Geometry check sheet. Reference: the model listing, model coordinates, mm. A direction names the side the tool comes from. Round coordinates to 2 decimals unless told otherwise and drop trailing zeros. Order: outer loops, then holes, each group sorted by start corner. A loop starts at its lowest first (then second) coordinate and runs counter-clockwise, first axis right, second up. Notation, with made-up numbers: (6, -12) - (54, -12) arc R26 ccw to (54, 19) - close; hole circle Ø1 at (28, 23). An arc over 180 degrees is marked (long way). Return JSON: item names as keys, results as strings. Group by question number.
Q1. Tool access check on faces 1 (the cylindrical face through (-36.39, -0.89, 4.93)), 2 (the cylindrical face through (24.245, -7.269, 25.196)), 3 (the cylindrical face through (29.14, 13.64, 21.3)). Record the directions out of +Z, -Z, +X, -X, +Y, -Y that give a thin tool (end or side, any length) a straight path to the whole face; none if there is none.
Q2. Sectioned sample at A-A, the plane y = -7.5. Give the number of separate pieces and of enclosed holes in the cut face, then the cut area to 3 significant figures.
Q3. Draft check along Y on faces 4 (the flat face through (25, 8, 22.2)), 5 (the cylindrical face through (0.591, -3.994, 14.001)), 6 (the conical face through (35.3, -0.1, 17.6)), 7 (the flat face through (16.7, -9.8, 6.5)). Enter one of: pulls with the +Y half, pulls with the -Y half, needs draft (parallel to the pull), parting line crosses it, or undercut.
Q4. Sectioned sample at B-B, the plane x = -18. Record the cut outline in (y, z).
Q5. Gauge pin test, flat ends, axial feed: pin 1 Ø5 at (x, y) = (20.5, -8) entering from -Z; pin 2 Ø1 at (x, z) = (2, 12) entering from +Y; pin 3 Ø8 at (x, z) = (4.5, 17.5) entering from +Y; pin 4 Ø5.5 at (x, y) = (-34.5, 14.48) entering from -Z. Record the tip position at first contact, or that the pin passes through.
Q6. Material ranges on line 1 along X through (y, z) = (-7.25, 18.2); line 2 along Y through (x, z) = (-19, 15.5); line 3 along Y through (x, z) = (-35, 3.5), recorded low to high.
Q7. Sectioned sample at C-C, the plane x = 25.5. Record the cut outline in (y, z).
Q8. Sectioned sample at D-D, the plane z = 24.5. Record the cut outline in (x, y).
```python
from build123d import *

# Parameters (mm, degrees)
EXTRUDE_1_DEPTH             = 28.4
SKETCH_2_W                  = 140
SKETCH_2_H                  = 16
CUT_EXTRUDE_1_DEPTH         = 20
FILLET_1_R                  = 3
SKETCH_3_R                  = 3
SKETCH_3_R_2                = 3.05
CUT_EXTRUDE_2_DEPTH         = 56.996071341
CHAMFER_1_SIZE              = 0.5
SKETCH_4_R                  = 3
CUT_EXTRUDE_3_DEPTH         = 55.394944713
SKETCH_7_R                  = 4.15
CUT_EXTRUDE_4_DEPTH         = 18
HOLE_WIZARD_M6_2_D          = 5
SKETCH_10_R                 = 3.1
CUT_EXTRUDE_5_DEPTH         = 55.394944713
HOLE_WIZARD_M5_1_D          = 4.2
HOLE_WIZARD_M5_1_DEPTH      = 14.4
HOLE_WIZARD_M5_1_TIP        = 1.2618073
HOLE_WIZARD_M5_2_D          = 4.2
HOLE_WIZARD_M5_2_DEPTH      = 14.4
HOLE_WIZARD_M5_2_TIP        = 1.2618073
FILLET_2_R                  = 1
SKETCH_17_R                 = 5.25
CUT_EXTRUDE_7_DEPTH         = 6.5
HOLE_WIZARD_M4_1_AT_2_COUNT = 2
HOLE_WIZARD_M4_1_AT_2_PITCH = 70
HOLE_WIZARD_M4_1_AT_3_COUNT = 2
HOLE_WIZARD_M4_1_AT_3_PITCH = 39.588508434


with BuildPart() as part:
    # 草图1 → 凸台-拉伸1 (new body)
    with BuildSketch(Plane.XY):
        with BuildLine():
            Line((27.5, 23.5), (40, 23.5))
            Line((40, 23.5), (40, -23.5))
            Line((40, -23.5), (-40, -23.5))
            Line((-40, -23.5), (-40, 23.5))
            Line((-40, 23.5), (-27.5, 23.5))
            ThreePointArc((-27.5, 23.5), (0, -4), (27.5, 23.5))
        make_face()
    extrude(amount=EXTRUDE_1_DEPTH)

    # 草图2 → 切除-拉伸1 (cut)
    with BuildSketch(Plane(origin=(0, 23.5, 0), x_dir=(1, 0, 0), z_dir=(0, 1, 0))):
        with Locations((-40, -14.2)):
            Rectangle(SKETCH_2_W, SKETCH_2_H)
    extrude(amount=-CUT_EXTRUDE_1_DEPTH, mode=Mode.SUBTRACT)

    # 圆角1
    # the kernel refuses this fillet: 3 mm, written as the material it adds along each edge
    with BuildSketch(Plane(origin=(30, 23.5, 22.2), x_dir=(-1, 0, 0), z_dir=(0, -1, 0))) as fillet_1_piece_1_section:
        with BuildLine():
            CenterArc((FILLET_1_R, FILLET_1_R), FILLET_1_R, 180, 90)
            Line((0, FILLET_1_R), (0, 0))
            Line((0, 0), (FILLET_1_R, 0))
        make_face()
    fillet_1_piece_1 = extrude(amount=27.5, mode=Mode.PRIVATE)
    fillet_1_piece_1 = fillet_1_piece_1 - Plane(origin=(0, 23.5, 21.518950585), x_dir=(-1, 0, 0), z_dir=(0, 0, -1)) * Cylinder(27.5, 67, mode=Mode.PRIVATE)
    add(fillet_1_piece_1)
    with BuildSketch(Plane(origin=(30, 23.5, 6.2), x_dir=(0, 0, 1), z_dir=(0, -1, 0))) as fillet_1_piece_2_section:
        with BuildLine():
            CenterArc((FILLET_1_R, FILLET_1_R), FILLET_1_R, 180, 90)
            Line((0, FILLET_1_R), (0, 0))
            Line((0, 0), (FILLET_1_R, 0))
        make_face()
    fillet_1_piece_2 = extrude(amount=27.5, mode=Mode.PRIVATE)
    fillet_1_piece_2 = fillet_1_piece_2 - Plane(origin=(0, 23.5, 6.881049416), x_dir=(-1, 0, 0), z_dir=(0, 0, -1)) * Cylinder(27.5, 68, mode=Mode.PRIVATE)
    add(fillet_1_piece_2)

    # 草图3 → 切除-拉伸2 (cut, through all)
    with BuildSketch(Plane(origin=(0, 3.5, 0), x_dir=(1, 0, 0), z_dir=(0, 1, 0))):
        with Locations(Location((-25.5, -10.2, 0), (0, 0, 270))):
            Circle(SKETCH_3_R)
        with Locations(Location((-25.5, -18.2, 0), (0, 0, 90))):
            Circle(SKETCH_3_R)
        with Locations(Location((25.5, -10.2, 0), (0, 0, 270))):
            Circle(SKETCH_3_R_2)
        with Locations(Location((25.5, -18.2, 0), (0, 0, 90))):
            Circle(SKETCH_3_R_2)
    extrude(amount=-CUT_EXTRUDE_2_DEPTH, mode=Mode.SUBTRACT)

    # 倒角1
    chamfer_1_edges = [part.edges().sort_by_distance(p)[0] for p in [
        (-25.5, 3.5, 7.2),
        (-25.5, 3.5, 21.2),
        (25.5, 3.5, 7.15),
        (25.5, 3.5, 21.25),
    ]]
    chamfer(chamfer_1_edges, length=CHAMFER_1_SIZE)

    # 草图4 → 切除-拉伸3 (cut, through all)
    with BuildSketch(Plane.XY.offset(28.4)):
        with Locations((-34.499379308, 14.475094051)):
            Circle(SKETCH_4_R)
    extrude(amount=-CUT_EXTRUDE_3_DEPTH, mode=Mode.SUBTRACT)

    # 草图7 → 切除-拉伸4 (cut)
    with BuildSketch(Plane(origin=(0, 23.5, 0), x_dir=(1, 0, 0), z_dir=(0, 1, 0))):
        with Locations(Location((35.2, -14.155033758, 0), (0, 0, 180))):
            Circle(SKETCH_7_R)
    extrude(amount=-CUT_EXTRUDE_4_DEPTH, mode=Mode.SUBTRACT)

    # M6 螺纹孔2 (through all)
    with Locations(Plane(origin=(0, 5.5, 0), x_dir=(1, 0, 0), z_dir=(0, 1, 0))):
        with Locations((35.2, -14.155033758)):
            Hole(HOLE_WIZARD_M6_2_D / 2)

    # 草图10 → 切除-拉伸5 (cut, through all)
    with BuildSketch(Plane.XY.offset(28.4)):
        with Locations((-19, -7.5)):
            Circle(SKETCH_10_R)
        with Locations(Location((19, -7.5, 0), (0, 0, 180))):
            Circle(SKETCH_10_R)
    extrude(amount=-CUT_EXTRUDE_5_DEPTH, mode=Mode.SUBTRACT)

    # M5 螺纹孔1
    with Locations(Plane.XY.offset(28.4)):
        with Locations((0, -11.5)):
            Hole(HOLE_WIZARD_M5_1_D / 2, depth=HOLE_WIZARD_M5_1_DEPTH)
            with Locations((0, 0, -(HOLE_WIZARD_M5_1_DEPTH + HOLE_WIZARD_M5_1_TIP / 2))):  # 118° drill point
                Cone(0, HOLE_WIZARD_M5_1_D / 2, HOLE_WIZARD_M5_1_TIP, mode=Mode.SUBTRACT)

    # M5 螺纹孔2
    with Locations(Plane(origin=(0, 0, 0), x_dir=(-1, 0, 0), z_dir=(0, 0, -1))):
        with Locations((0, -11.5)):
            Hole(HOLE_WIZARD_M5_2_D / 2, depth=HOLE_WIZARD_M5_2_DEPTH)
            with Locations((0, 0, -(HOLE_WIZARD_M5_2_DEPTH + HOLE_WIZARD_M5_2_TIP / 2))):  # 118° drill point
                Cone(0, HOLE_WIZARD_M5_2_D / 2, HOLE_WIZARD_M5_2_TIP, mode=Mode.SUBTRACT)

    # 圆角2
    fillet_2_edges = [part.edges().sort_by_distance(p)[0] for p in [
        (27.5, 23.5, 25.279019946),
        (27.5, 23.5, 3.120980054),
        (-27.5, 23.5, 25.3),
        (-27.5, 23.5, 3.1),
    ]]
    fillet(fillet_2_edges, radius=FILLET_2_R)

    # 草图17 → 切除-拉伸7 (cut)
    with BuildSketch(Plane(origin=(0, 0, 0), x_dir=(-1, 0, 0), z_dir=(0, 0, -1))):
        with Locations((-19, -7.5)):
            Circle(SKETCH_17_R)
        with Locations((19, -7.5)):
            Circle(SKETCH_17_R)
    cut_extrude_7 = extrude(amount=-CUT_EXTRUDE_7_DEPTH, mode=Mode.SUBTRACT)

    # 镜向3: 切除-拉伸7 across plane
    add(cut_extrude_7.mirror(Plane.XY.offset(14.2)), mode=Mode.SUBTRACT)

    # 草图18 → M4 螺纹孔1 (revolve, cut)
    with BuildSketch(Plane(origin=(-35, 0, 28.4), x_dir=(0, -1, 0), z_dir=(1, 0, 0))):
        Polygon((0, 0), (0, 10.991420021), (1.65, 10), (1.65, 0), align=None)
    hole_wizard_m4_1 = revolve(axis=Axis((-35, 0, 34.75), (0, 0, -1)), mode=Mode.SUBTRACT)

    # M4 螺纹孔1 at 2: M4 螺纹孔1 ×2
    with Locations(*[(i * HOLE_WIZARD_M4_1_AT_2_PITCH, 0, 0) for i in range(1, HOLE_WIZARD_M4_1_AT_2_COUNT)]):
        add(hole_wizard_m4_1, mode=Mode.SUBTRACT)

    # M4 螺纹孔1 at 3: M4 螺纹孔1 ×2
    with Locations(*[Vector(0.8840949402949304, -0.46730732558446325, 0) * (i * HOLE_WIZARD_M4_1_AT_3_PITCH) for i in range(1, HOLE_WIZARD_M4_1_AT_3_COUNT)]):
        add(hole_wizard_m4_1, mode=Mode.SUBTRACT)

    # 镜向4: M4 螺纹孔1 across plane
    add(hole_wizard_m4_1.mirror(Plane.XY.offset(14.2)), mode=Mode.SUBTRACT)

    # 镜向4 copy 1 sketch → 镜向4 copy 1 (revolve, cut)
    with BuildSketch(Plane(origin=(35, 0, 0), x_dir=(0, -1, 0), z_dir=(1, 0, 0))):
        Polygon((0, 0), (0, -10.991420021), (1.65, -10), (1.65, 0), align=None)
    revolve(axis=Axis((35, 0, -6.35), (0, 0, -1)), mode=Mode.SUBTRACT)

    # 镜向4 copy 2 sketch → 镜向4 copy 2 (revolve, cut)
    with BuildSketch(Plane(origin=(0, -18.5, 0), x_dir=(0, -1, 0), z_dir=(1, 0, 0))):
        Polygon((0, 0), (0, -10.991420021), (1.65, -10), (1.65, 0), align=None)
    revolve(axis=Axis((0, -18.5, -6.35), (0, 0, -1)), mode=Mode.SUBTRACT)


solid = part.part
```
Reply:
{
 "1": {"face 1": "-Z", "face 2": "+Z", "face 3": "-X, +Y"},
 "2": {"separate pieces": "3", "enclosed holes": "5", "area": "1,670 mm^2"},
 "3": {"face 4": "needs draft", "face 5": "pulls with the +Y half", "face 6": "undercut", "face 7": "undercut"},
 "4": {"outline": "(-23.5, 0) - (-12.65, 0) - (-12.65, 6.5) - (-10.43, 6.5) - (-10.43, 21.9) - (-12.65, 21.9) - (-12.65, 28.4) - (-23.5, 28.4) - close; (-4.57, 6.5) - (-2.35, 6.5) - (-2.35, 0) - (2.71, 0) - (2.71, 28.4) - (-2.35, 28.4) - (-2.35, 21.9) - (-4.57, 21.9) - close"},
 "5": {"pin 1": "z = 6.5", "pin 2": "y = -3.89", "pin 3": "y = -2.65", "pin 4": "through"},
 "6": {"line 1": "-40 to -28.5, -22.5 to -22.09, -15.91 to 15.91, 22.09 to 22.45, 28.55 to 40", "line 2": "-23.5 to -10.6, -4.4 to 3.5", "line 3": "-23.5 to -1.65, 1.65 to 11.52, 17.43 to 23.5"},
 "7": {"outline": "(-23.5, 0) - (13.2, 0) - (13.2, 6.2) - (3.5, 6.2) - (3.5, 6.65) - (3, 7.15) - (-23.5, 7.15) - close; (-23.5, 13.25) - (3, 13.25) - (3.5, 13.75) - (3.5, 14.65) - (3, 15.15) - (-23.5, 15.15) - close; (-23.5, 21.25) - (3, 21.25) - (3.5, 21.75) - (3.5, 22.2) - (13.2, 22.2) - (13.2, 28.4) - (-23.5, 28.4) - close"},
 "8": {"outline": "(-40, -23.5) - (40, -23.5) - (40, 23.5) - (28.48, 23.5) arc R1 ccw to (27.48, 22.54) arc R27.5 cw to (-27.48, 22.54) arc R1 ccw to (-28.48, 23.5) - (-40, 23.5) - close; hole circle Ø6 at (-34.5, 14.48); hole circle Ø3.3 at (-35, 0); hole circle Ø10.5 at (-19, -7.5); hole circle Ø4.2 at (0, -11.5); hole circle Ø3.3 at (0, -18.5); hole circle Ø10.5 at (19, -7.5); hole circle Ø3.3 at (35, 0)"}
}
